from build123d import *

# Parameters (mm, degrees)
F0_W     = 62.8466829658
F0_H     = 52.6766888797
F1_DEPTH = 6
F2_W     = 13.9663396403
F2_H     = 11.3499658182
F3_DEPTH = 63
F4_W     = 11.3499658182
F4_H     = 11.0394264162
F5_DEPTH = 28
F6_W     = 13.0074043497
F6_H     = 11.0394264162
F7_DEPTH = 43
F8_W     = 11.1150065735
F8_H     = 11.0394264162
F9_DEPTH = 24


with BuildPart() as f1:
    # F0 (on Top) → F1 (new body)
    with BuildSketch(Plane.XY):
        with Locations((2.4644061923, -3.5718083382)):
            Rectangle(F0_W, F0_H)
    extrude(amount=F1_DEPTH)

    # F2 (on face) → F3 (join)
    with BuildSketch(Plane.XY.offset(6)):
        with Locations((-21.9757654704, 17.0915531926)):
            Rectangle(F2_W, F2_H)
    extrude(amount=F3_DEPTH)

    # F4 (on face) → F5 (join)
    with BuildSketch(Plane.YZ.offset(-14.9925956503)):
        with Locations((17.0915531926, 63.4802867919)):
            Rectangle(F4_W, F4_H)
    extrude(amount=F5_DEPTH)

    # F6 (on face) → F7 (join)
    with BuildSketch(Plane.XZ.offset(-11.4165702835)):
        with Locations((6.5037021749, 63.4802867919)):
            Rectangle(F6_W, F6_H)
    extrude(amount=F7_DEPTH)

    # F8 (on face) → F9 (join)
    with BuildSketch(Plane.YZ.offset(13.0074043497)):
        with Locations((-26.0259264298, 63.4802867919)):
            Rectangle(F8_W, F8_H)
    extrude(amount=F9_DEPTH)


solid = f1.part
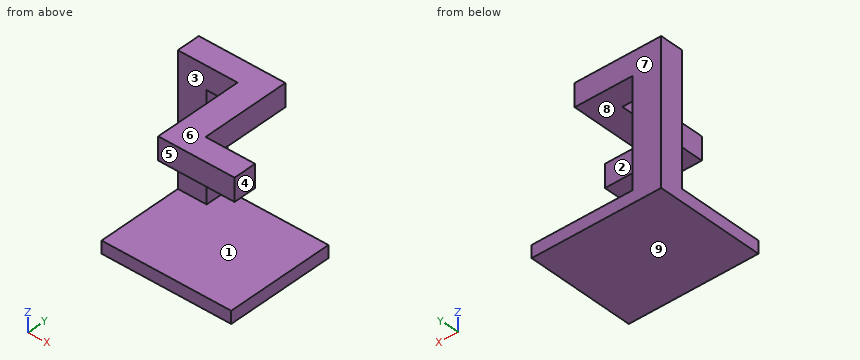
Work out the finished part from the listing and answer in its coordinate system (mm). Face numbers are marked on the shaded views. A direction names the side the tool comes from. Give positions to 0.01 mm unless a question says otherwise; leave off trailing zeros. Write each loop counter-clockwise with the first axis right and the second up, starting at its lowest first coordinate (ties: lowest second). Pieces come first, ordered by that corner, then holes. Notation, with made-up numbers: (23, 67.25) - (71, 67.25) arc R6 ccw to (71, 76.25) - close; hole circle Ø3 at (14, 70). An arc over 180 degrees is marked (long way). One line per item, written item: value. Start each with the question number.
1. For a pull along Z with two mould halves and no side action, classify the marked faces 6, 7, 8 and 9 as +Z half, -Z half, draft (parallel to the pull), parting line (faces both ways), or undercut.
2. For the marked faces 1, 2, 3, 4 and 5, determine the directions among +Z, -Z, +X, -X, +Y, -Y from which every point of the face is accessible in a straight line to the end or side of a thin tool.
3. Find section D-D (y = 18.5). Write down the section's boundary in (x, z).
4. Find section A-A (x = 6). Write down the section's boundary in (y, z), then the cut area to 3 significant figures.
5. Find section B-B (y = 10). Write down the section's boundary in (x, z).
6. Find section C-C (z = 63.5). Write down the section's boundary in (x, y).
7. Consider probe 1 along Z at (x, y) = (-14, 20); probe 2 along Y at (x, z) = (-20.5, 65); probe 3 along Z at (x, y) = (17, 5). Determine where each line is inside the solid, lowest interval first.
8. Given pin 1 (9 mm diameter, centred on y = 3, z = 62, fed in from +X); pin 2 (9 mm diameter, centred on x = 28.5, z = 65.5, fed in from +Y); pin 3 (9 mm diameter, centred on y = -5, z = 63.5, fed in from -X), each flat-ended and moving along its own axis, determine where each tip first touches the part or whether it passes through.
Geometry results:
1. face 6: +Z half
1. face 7: draft
1. face 8: undercut
1. face 9: -Z half
2. face 1: +X, -Y
2. face 2: +Z, +X, +Y
2. face 3: +Z, -X, -Y
2. face 4: +Z, -Z, +X, +Y, -Y
2. face 5: +Z, -Z, +X, -X, -Y
3. outline: (-28.96, 0) - (33.89, 0) - (33.89, 6) - (-14.99, 6) - (-14.99, 57.96) - (13.01, 57.96) - (13.01, 69) - (-28.96, 69) - close
4. outline: (-31.58, 57.96) - (22.77, 57.96) - (22.77, 69) - (-31.58, 69) - close; (-29.91, 0) - (22.77, 0) - (22.77, 6) - (-29.91, 6) - close
4. area: 916 mm2
5. outline: (-28.96, 0) - (33.89, 0) - (33.89, 6) - (-28.96, 6) - close; (0, 57.96) - (13.01, 57.96) - (13.01, 69) - (0, 69) - close
6. outline: (-28.96, 11.42) - (0, 11.42) - (0, -31.58) - (37.01, -31.58) - (37.01, -20.47) - (13.01, -20.47) - (13.01, 22.77) - (-28.96, 22.77) - close
7. probe 1: 0 to 6, 57.96 to 69
7. probe 2: 11.42 to 22.77
7. probe 3: 0 to 6
8. pin 1: x = 13.01
8. pin 2: y = -20.47
8. pin 3: x = 0
